Source: CAD feature listing. Evaluate the final solid. Frame: model axes, mm. Give positions to 0.01 mm unless a question says otherwise; leave off trailing zeros. Loops run counter-clockwise (first coordinate to the right, second up) from the corner with the lowest first, then second, coordinate; pieces in that order, holes last. Notation, with made-up numbers: M -11.75,-26 L 19.25,-26 A36 ccw 19.25,12 Z; hole C 22,5 d8. An arc over 180 degrees is marked long. Answer in a Markdown table with one row per item.
Autodesk Inventor part; units mm, degrees
ref_plane "YZ Plane" through (0, 0, 0) normal (1, 0, 0) x (0, 1, 0)
ref_plane "XZ Plane" through (0, 0, 0) normal (0, 1, 0) x (-1, 0, 0)
ref_plane "XY Plane" through (0, 0, 0) normal (0, 0, 1) x (1, 0, 0)
sketch "Sketch1" plane through (0, 0, 0) normal (0, 0, 1) x (1, 0, 0)
  line L0 (-0.7792, 0.974) -> (1.2208, 0.974)
  line L1 (1.2208, 0.974) -> (1.2208, -1.026)
  line L2 (1.2208, -1.026) -> (-0.7792, -1.026)
  line L3 (-0.7792, -1.026) -> (-0.7792, 0.974)
  point P0 (0, 0)
  dimension "d0" = 2
extrude "Extrusion1" add sketch "Sketch1" along normal blind 20
fillet "Fillet1" radius 0.889 4 edges at (-0.7792, -0.026, 20) (1.2208, -0.026, 20) (1.2208, -0.026, 0) (-0.7792, -0.026, 0)
properties part number "Maybe CIM Key"
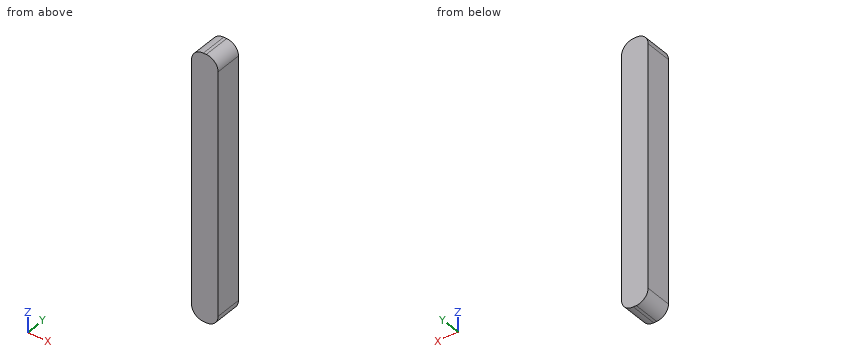
1) Section B-B, the plane x = 1. Return loops of the section in (y, z), then the cut area to 3 significant figures.
Reply:
| item | result |
|---|---|
| outline | M -1.03,0.3 L 0.97,0.3 L 0.97,19.7 L -1.03,19.7 Z |
| area | 38.8 mm² |
2) Material intervals for L1, parallel to Z at x = 0.4, y = -0.8; L2, parallel to Z at x = 1.1, y = 0.6, sorted ascending.
Reply:
| item | result |
|---|---|
| L1 | z = 0 to 20 |
| L2 | z = 0.44 to 19.56 |
3) Section A-A, the plane y = -0.55. Return loops of the section in (x, z).
Reply:
| item | result |
|---|---|
| outline | M -0.78,0.89 A0.89 ccw 0.11,0 L 0.33,0 A0.89 ccw 1.22,0.89 L 1.22,19.11 A0.89 ccw 0.33,20 L 0.11,20 A0.89 ccw -0.78,19.11 Z |
